from build123d import *

# Parameters (mm, degrees)
F0_W     = 184.15
F0_H     = 101.6
F1_DEPTH = 12.7
F3_D     = 12.7
F5_D     = 7.9375
F7_D     = 7.9375


with BuildPart() as f1:
    # F0 (on Front) → F1 (new body)
    with BuildSketch(Plane.XZ):
        with Locations((92.075, 50.8)):
            Rectangle(F0_W, F0_H)
    extrude(amount=F1_DEPTH)

    # F3 (through all)
    with Locations(Plane.XZ.offset(12.7)):
        with Locations((92.075, 76.2)):
            Hole(F3_D / 2)

    # F5 (through all)
    with Locations(Plane.XZ.offset(12.7)):
        with Locations((22.225, 63.5), (161.925, 63.5), (161.925, 12.7), (22.225, 12.7)):
            Hole(F5_D / 2)

    # F7 (through all)
    with Locations(Plane.XZ.offset(12.7)):
        with Locations((41.275, 31.75), (142.875, 31.75), (30.1625, 31.75), (153.9875, 31.75)):
            Hole(F7_D / 2)


solid = f1.part
The listing builds one solid part. Answer for the finished solid, in the listing's coordinates (mm). Give positions to 0.01 mm unless a question says otherwise; leave off trailing zeros. Order: outer loops, then holes, each group sorted by start corner. A loop starts at its lowest first (then second) coordinate and runs counter-clockwise, first axis right, second up. Notation, with made-up numbers: (-4.5, 45) - (36.5, 45) arc R22 cw to (36.5, 67) - close; hole circle Ø10 at (24, -37). An arc over 180 degrees is marked (long way). One line per item, written item: value. Start each with the question number.
1) A cutting plane is placed at D-D on x = 162. Give the vertices of the cut face in (y, z).
2) A cutting plane is placed at B-B on y = -5.75. State how many separate pieces and enclosed holes the cut face has, then the cut area to 3 significant figures.
3) A cutting plane is placed at C-C on z = 31.75. Give the vertices of the cut face in (x, y), then the cut area to 3 significant figures.
4) Find the intervals of material crossed by L1, parallel to X at y = -1.75, z = 32; L2, parallel to X at y = -9.5, z = 16; L3, parallel to X at y = -3, z = 75.5, in increasing order.
5) The mould has two halves that part along Z. Classify faces 1 (the face through (91, -6, 0)), 2 (the face through (146.024, -6.261, 29.335)), 3 (the face through (91, 0, 52)), 4 (the face through (22.742, -6.261, 67.435)): released by +Z, released by -Z, zero draft, split by the parting line, or undercut.
6) A cutting plane is placed at A-A on z = 76.2. Give the vertices of the cut face in (x, y) (3 decimals), then the cut area to 3 significant figures.
Answer sheet:
1. outline: (-12.7, 0) - (0, 0) - (0, 8.73) - (-12.7, 8.73) - close; (-12.7, 16.67) - (0, 16.67) - (0, 59.53) - (-12.7, 59.53) - close; (-12.7, 67.47) - (0, 67.47) - (0, 101.6) - (-12.7, 101.6) - close
2. separate pieces: 1
2. enclosed holes: 9
2. area: 18,200 mm2
3. outline: (0, -12.7) - (26.19, -12.7) - (26.19, 0) - (0, 0) - close; (34.13, -12.7) - (37.31, -12.7) - (37.31, 0) - (34.13, 0) - close; (45.24, -12.7) - (138.91, -12.7) - (138.91, 0) - (45.24, 0) - close; (146.84, -12.7) - (150.02, -12.7) - (150.02, 0) - (146.84, 0) - close; (157.96, -12.7) - (184.15, -12.7) - (184.15, 0) - (157.96, 0) - close
3. area: 1,940 mm2
4. L1: x = 0 to 26.2, 34.12 to 37.31, 45.24 to 138.91, 146.84 to 150.03, 157.95 to 184.15
4. L2: x = 0 to 20.02, 24.43 to 159.72, 164.13 to 184.15
4. L3: x = 0 to 85.76, 98.39 to 184.15
5. face 1: released by -Z
5. face 2: undercut
5. face 3: zero draft
5. face 4: undercut
6. outline: (0, -12.7) - (85.725, -12.7) - (85.725, 0) - (0, 0) - close; (98.425, -12.7) - (184.15, -12.7) - (184.15, 0) - (98.425, 0) - close
6. area: 2,180 mm2
